```python
from build123d import *

# Parameters (mm, degrees)
F0_R     = 31.75
F0_R_2   = 10
F1_DEPTH = 290
F2_DEPTH = 76.2
F3_R     = 10
F4_DEPTH = 76.2
F5_R     = 2.5
F5_R_2   = 2.5019
F6_DEPTH = 63.5


with BuildPart() as f1:
    # F0 (on Front) → F1 (new body)
    with BuildSketch(Plane.XZ):
        Circle(F0_R)
        Circle(F0_R_2, mode=Mode.SUBTRACT)
        Circle(F0_R_2)
    extrude(amount=-F1_DEPTH)

    # F0 (on Front) → F2 (join)
    with BuildSketch(Plane.XZ):
        Circle(F0_R_2)
    extrude(amount=F2_DEPTH)

    # F3 (on face) → F4 (join)
    with BuildSketch(Plane(origin=(0, 290, 0), x_dir=(-1, 0, 0), z_dir=(0, 1, 0))):
        Circle(F3_R)
    extrude(amount=F4_DEPTH)

    # F5 (on Right) → F6 (cut, symmetric)
    with BuildSketch(Plane.YZ):
        with Locations((-64.77, 0)):
            Circle(F5_R)
        with Locations((354.77, 0)):
            Circle(F5_R_2)
    extrude(amount=F6_DEPTH, both=True, mode=Mode.SUBTRACT)


solid = f1.part
```
Work out the finished part from the listing and answer in its coordinate system (mm). A direction names the side the tool comes from. Coordinates: 2 decimals unless noted, no trailing zeros. Loops run counter-clockwise (first coordinate to the right, second up) from the corner with the lowest first, then second, coordinate; pieces in that order, holes last. Notation, with made-up numbers: (-14, -21) -> (8, -21) arc R27 ccw to (8, 4) -> close; hole circle Ø9 at (-5, 62.5). An arc over 180 degrees is marked (long way). Answer as CSV lines item,"result".
Q1. The part is cut by section A-A on x = -4. Write down the section's boundary in (y, z).
Findings:
outline,"(-76.2, -9.17) -> (0, -9.17) -> (0, -31.5) -> (290, -31.5) -> (290, -9.17) -> (366.2, -9.17) -> (366.2, 9.17) -> (290, 9.17) -> (290, 31.5) -> (0, 31.5) -> (0, 9.17) -> (-76.2, 9.17) -> close; hole circle Ø5 at (-64.77, 0); hole circle Ø5 at (354.77, 0)"
Q2. The part is cut by section C-C on z = -25.5. Write down the section's boundary in (x, y), and give its area (3 significant figures).
Findings:
outline,"(-18.92, 0) -> (18.92, 0) -> (18.92, 290) -> (-18.92, 290) -> close"
area,"11,000 mm²"
Q3. The part is cut by section D-D on y = 211.5. Write down the section's boundary in (x, z).
Findings:
outline,"circle Ø63.5 at (0, 0)"
Q4. The part is cut by section B-B on y = -42. Write down the section's boundary in (x, z), and give its area (3 significant figures).
Findings:
outline,"circle Ø20 at (0, 0)"
area,"314 mm²"
Q5. A tool of negligible diameter and unlimited length cuts with its end or side. For faces 1 (the face through (0, 366.2, 0)), 2 (the face through (-8, 290, 8)), 3 (the face through (-8, 0, 8)), from which of +Z, -Z, +X, -X, +Y, -Y can it reach the whole face along a straight path? Write none if from no direction.
Findings:
face 1,"+Z, -Z, +X, -X, +Y"
face 2,"+Y"
face 3,"-Y"
Q6. Each of these flat-tipped pins is pushed along its axis until it touches: pin 1 (12 mm diameter, centred on x = -25, z = 0.5, fed in from -Y); pin 2 (2 mm diameter, centred on x = 17.5, y = 3, fed in from -Z); pin 3 (10 mm diameter, centred on y = 128, z = -17.5, fed in from -X); pin 4 (4.5 mm diameter, centred on y = -64.77, z = 0, fed in from -X). Where does it stop, or does it pass through?
Findings:
pin 1,"stops at y = 0"
pin 2,"stops at z = -27.13"
pin 3,"stops at x = -29.19"
pin 4,"passes through"
Q7. Find the intervals of material crossed by probe 1 along Y at (x, z) = (-7.25, 0); probe 2 along Y at (x, z) = (-4.5, -27); probe 3 along Z at (x, y) = (2.5, -64.77), in increasing order.
Findings:
probe 1,"y = -76.2 to -67.27, -62.27 to 352.27, 357.27 to 366.2"
probe 2,"y = 0 to 290"
probe 3,"z = -9.68 to -2.5, 2.5 to 9.68"
